Geometry: final body of the model. Coordinates: model frame, mm. Face numbers are marked on the shaded views. A direction names the side the tool comes from. Give positions to 0.01 mm unless a question says otherwise; leave off trailing zeros. Write each loop counter-clockwise with the first axis right and the second up, starting at its lowest first coordinate (ties: lowest second). Pieces come first, ordered by that corner, then holes.
from build123d import *

# Parameters (mm, degrees)
F0_R     = 6
F1_DEPTH = 20
F2_DEPTH = 10
F4_DEPTH = 25
F5_R     = 1


with BuildPart() as f1:
    # F0 (on Top) → F1 (new body)
    with BuildSketch(Plane.XY):
        Circle(F0_R)
        with BuildLine():
            ThreePointArc((-2.525, 1.841195), (3.125, 0), (-2.525, -1.841195))
            Line((-2.525, -1.841195), (-2.525, 1.841195))
        make_face(mode=Mode.SUBTRACT)
    extrude(amount=F1_DEPTH)

    # F0 (on Top) → F2 (join)
    with BuildSketch(Plane.XY):
        with BuildLine():
            Line((-2.525, 1.841195), (-2.525, -1.841195))
            ThreePointArc((-2.525, -1.841195), (3.125, 0), (-2.525, 1.841195))
        make_face()
    extrude(amount=F2_DEPTH)

    # F3 (on face) → F4 (cut)
    with BuildSketch(Plane(origin=(0, 0, 0), x_dir=(1, 0, 0), z_dir=(0, 0, -1))):
        with BuildLine():
            Line((-2.1, 1.356466), (-2.1, -1.356466))
            ThreePointArc((-2.1, -1.356466), (2.5, 0), (-2.1, 1.356466))
        make_face()
    extrude(amount=-F4_DEPTH, mode=Mode.SUBTRACT)

    # F5
    f5_edges = [f1.edges().sort_by_distance(p)[0] for p in [
        (-6, 0, 20),
        (-6, 0, 0),
    ]]
    fillet(f5_edges, radius=F5_R)


solid = f1.part
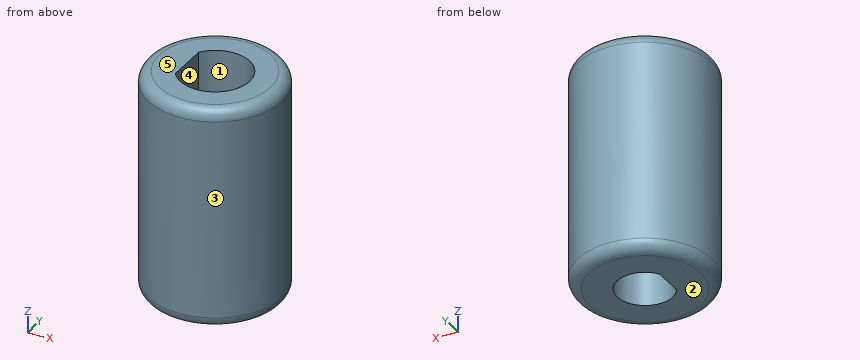
Q1. Section A-A on x = 0. Output: boundary loops of the cut face in (y, z) (3 decimals).
Filled sheet:
outline: (-6, 1) arc R1 ccw to (-5, 0) - (-2.5, 0) - (-2.5, 10) - (-3.125, 10) - (-3.125, 20) - (-5, 20) arc R1 ccw to (-6, 19) - close; (2.5, 0) - (5, 0) arc R1 ccw to (6, 1) - (6, 19) arc R1 ccw to (5, 20) - (3.125, 20) - (3.125, 10) - (2.5, 10) - close
Q2. Pin query (flat end, axial travel): P1, Ø3, axis at x = -3, z = 11, coming from the +Y side; P2, Ø6, axis at y = -3.5, z = 11.5, coming from the -X side; P3, Ø1.1, axis at y = -0.5, z = 12.5, coming from the +X side; P4, Ø4.5, axis at x = 0, y = 0, coming from the +Z side. Return the tip coordinate at first contact, or that it passes through.
Filled sheet:
P1: stops at y = 5.81
P2: stops at x = -5.98
P3: stops at x = 6
P4: stops at z = 10
Q3. Section C-C on z = 10.5. Output: boundary loops of the cut face in (x, y) (3 decimals).
Filled sheet:
outline: circle Ø12 at (0, 0); hole (-2.525, -1.841) arc R3.125 ccw (long way) to (-2.525, 1.841) - close
Q4. Access query for the marked faces 1 and 2. Directions: +Z, -Z, +X, -X, +Y, -Y. A direction counts if a zero-diameter tool reaches every point of the face in a straight line with its end or side. Return the directions, or none.
Filled sheet:
face 1: +Z
face 2: -Z, +X, -X, +Y, -Y
Q5. Section B-B on y = 0. Output: boundary loops of the cut face in (x, z) (3 decimals).
Filled sheet:
outline: (-6, 1) arc R1 ccw to (-5, 0) - (-2.1, 0) - (-2.1, 10) - (-2.525, 10) - (-2.525, 20) - (-5, 20) arc R1 ccw to (-6, 19) - close; (2.5, 0) - (5, 0) arc R1 ccw to (6, 1) - (6, 19) arc R1 ccw to (5, 20) - (3.125, 20) - (3.125, 10) - (2.5, 10) - close
Q6. Pull-direction query (X, two-part tool) for the marked faces 3, 4 and 5; classes: released by +X, released by -X, zero draft, split by the parting line, or undercut.
Filled sheet:
face 3: split by the parting line
face 4: undercut
face 5: zero draft
Q7. Ray query, line 1 along Y through (x, z) = (0, 15) (3 decimals); line 2 along Y through (x, z) = (0, 6.75); line 3 along Z through (x, y) = (5, 0.75). Return the intervals inside material, ascending.
Filled sheet:
line 1: y = -6 to -3.125, 3.125 to 6
line 2: y = -6 to -2.5, 2.5 to 6
line 3: z = 0 to 20
Q8. Section D-D on z = 8. Output: boundary loops of the cut face in (x, y), plus the area to 3 significant figures.
Filled sheet:
outline: circle Ø12 at (0, 0); hole (-2.1, -1.36) arc R2.5 ccw (long way) to (-2.1, 1.36) - close
area: 94.2 mm2
